```python
from build123d import *

# Parameters (mm, degrees)
SKETCH_1_W        = 5
SKETCH_1_H        = 10
EXTRUDE_1_DEPTH   = 7
EXTRUDE_1_2_DEPTH = 7
EXTRUDE_2_DEPTH   = 4


with BuildPart() as part:
    # Sketch 1 → Extrude 1 (new body)
    with BuildSketch(Plane(origin=(0, 0, 0), x_dir=(1, 0, 0), z_dir=(0, 1, 0))):
        with Locations((-39.97, 5)):
            Rectangle(SKETCH_1_W, SKETCH_1_H)
    extrude(amount=EXTRUDE_1_DEPTH)



with BuildPart() as body_2:
    # Sketch 1 → Extrude 1 2 (new body)
    with BuildSketch(Plane(origin=(0, 0, 0), x_dir=(1, 0, 0), z_dir=(0, 1, 0))):
        with Locations((39.97, 5)):
            Rectangle(SKETCH_1_W, SKETCH_1_H)
    extrude(amount=EXTRUDE_1_2_DEPTH)


with BuildPart() as part_1:
    add(part.part)

    add(body_2.part)  # Extrude 2 merges body 2
    # Sketch 2 → Extrude 2 (add)
    with BuildSketch(Plane(origin=(0, 7, 0), x_dir=(1, 0, 0), z_dir=(0, 1, 0))):
        Polygon((0, 26.25), (0, 29.7), (-26.47, 29.7), (-26.47, 26.25), (-23.47, 26.25), align=None)
        Polygon((-26.47, 26.25), (-26.47, 29.7), (-37.47, 10), (-37.47, 0), (-26.47, 7.7), (-26.47, 11.15), (-23.47, 11.15), (-23.47, 26.25), align=None)
        Polygon((26.47, 26.25), (26.47, 29.7), (0, 29.7), (0, 26.25), (23.47, 26.25), align=None)
        Polygon((23.47, 11.15), (0, 11.15), (0, 7.7), (26.47, 7.7), (26.47, 11.15), align=None)
        Polygon((0, 7.7), (0, 11.15), (-23.47, 11.15), (-26.47, 11.15), (-26.47, 7.7), align=None)
        Polygon((37.47, 10), (26.47, 29.7), (26.47, 26.25), (23.47, 26.25), (23.47, 11.15), (26.47, 11.15), (26.47, 7.7), (37.47, 0), align=None)
    extrude(amount=-EXTRUDE_2_DEPTH)


solid = part_1.part
```
The model under review builds one solid part; all positions refer to its coordinate system, in mm. A direction names the side the tool comes from. Give positions to 0.01 mm unless a question says otherwise; leave off trailing zeros. Write each loop counter-clockwise with the first axis right and the second up, starting at its lowest first coordinate (ties: lowest second). Pieces come first, ordered by that corner, then holes. Notation, with made-up numbers: M -22,31 L -11,31 A27 cw -11,69 Z; hole C 52.25,-35.75 d4. An arc over 180 degrees is marked long. Write item = value, one per line. Start each with the question number.
Q1. Mouldability with a two-part tool opening along Z and no side actions: class faces 5 (the face through (23.47, 5, -19)), 6 (the face through (32.05, 5.03, -19.71)), 7 (the face through (-37.47, 1, -5)), 8 (the face through (31.9, 5, -3.9)) as released by +Z, released by -Z, zero draft, split by the parting line, or undercut.
Q2. We need section C-C (z = -1.75). State the section outline as (x, y) points, plus the area to 3 significant figures.
Q3. Clearance check with flat-ended pins moving along their axes: pin 1 (2 mm diameter, centred on x = -0.5, y = 4.5, fed in from +Z); pin 2 (5 mm diameter, centred on x = -27.5, z = -11, fed in from -Y); pin 3 (1.2 mm diameter, centred on y = 5, z = -21, fed in from +X). State where each tip first meets the part, or that it passes through.
Q4. Machinability: for faces 1 (the face through (-32.047, 5.028, -3.796)), 2 (the face through (37.47, 1, -5)), 3 (the face through (-23.47, 5, -19)), 4 (the face through (-40, 3, -10)), which of the approach directions +Z, -Z, +X, -X, +Y, -Y give a long, thin tool a straight path to every point of the face, cutting with its end or side? Answer none if there is none.
Q5. We need section B-B (y = 2). State the section outline as (x, z) points.
Q6. For line 1 (X direction, y = 2.25, z = -3.5); line 2 (Z direction, x = -7.5, y = 6.25); line 3 (X direction, y = 5.25, z = -22.5), list the stretches that pass through material, from the lowest coordinate up.
Q7. We need section A-A (x = 12.5). State the section outline as (y, z) points, plus the area to 3 significant figures.
Q8. We need section D-D (z = -6.25). State the section outline as (x, y) points.
Result set:
q1.face_5 = undercut
q1.face_6 = released by -Z
q1.face_7 = zero draft
q1.face_8 = released by +Z
q2.outline = M -42.47,0 L -37.47,0 L -37.47,3 L -34.97,3 L -34.97,7 L -42.47,7 Z; M 34.97,3 L 37.47,3 L 37.47,0 L 42.47,0 L 42.47,7 L 34.97,7 Z
q2.area = 90.0 mm2
q3.pin_1 = -7.7
q3.pin_2 = 3
q3.pin_3 = 31.66
q4.face_1 = +Z, +Y, -Y
q4.face_2 = +Z, -Z, -Y
q4.face_3 = +Y, -Y
q4.face_4 = -Z, -X, +Y, -Y
q5.outline = M -42.47,-10 L -37.47,-10 L -37.47,0 L -42.47,0 Z; M 37.47,-10 L 42.47,-10 L 42.47,0 L 37.47,0 Z
q6.line_1 = -42.47 to -37.47, 37.47 to 42.47
q6.line_2 = -29.7 to -26.25, -11.15 to -7.7
q6.line_3 = -30.49 to -23.47, 23.47 to 30.49
q7.outline = M 3,-29.7 L 7,-29.7 L 7,-26.25 L 3,-26.25 Z; M 3,-11.15 L 7,-11.15 L 7,-7.7 L 3,-7.7 Z
q7.area = 27.6 mm2
q8.outline = M -42.47,0 L -37.47,0 L -37.47,3 L -28.54,3 L -28.54,7 L -42.47,7 Z; M 28.54,3 L 37.47,3 L 37.47,0 L 42.47,0 L 42.47,7 L 28.54,7 Z
